Geometry check sheet. Reference: the model listing, model coordinates, mm. Face numbers are marked on the shaded views. Coordinates: 2 decimals unless noted, no trailing zeros. Loops run counter-clockwise (first coordinate to the right, second up) from the corner with the lowest first, then second, coordinate; pieces in that order, holes last. Notation, with made-up numbers: (2.5, -27) -> (61.5, -27) arc R24 ccw to (61.5, 5) -> close; hole circle Ø7 at (7, 57). An arc over 180 degrees is marked (long way). Answer as a JSON object with one key per item and string values.
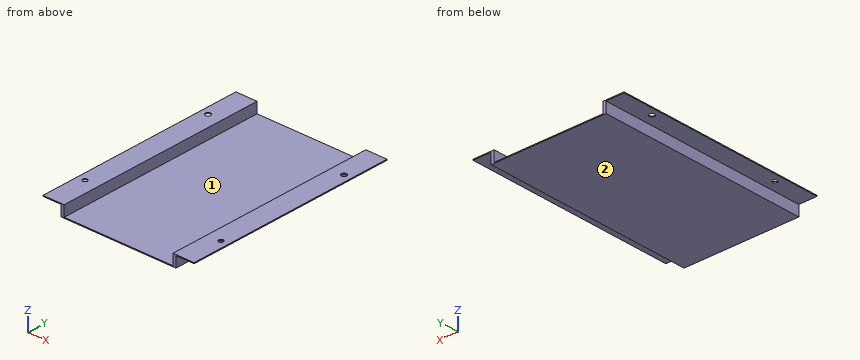
Autodesk Inventor part; units mm, degrees
ref_plane "YZ Plane" through (0, 0, 0) normal (1, 0, 0) x (0, 1, 0)
ref_plane "XZ Plane" through (0, 0, 0) normal (0, 1, 0) x (-1, 0, 0)
ref_plane "XY Plane" through (0, 0, 0) normal (0, 0, 1) x (1, 0, 0)
sketch "Skizze1" plane through (0, 0, 0) normal (0, 0, 1) x (1, 0, 0)
  line L0 (-90, 421.0534) -> (-90, 451.3884) construction
  line L1 (-90, 311.0534) -> (10, 311.0534)
  line L2 (10, 311.0534) -> (10, 451.0534)
  line L3 (10, 451.0534) -> (-90, 451.0534)
  line L4 (-90, 451.0534) -> (-90, 311.0534)
  circle A0 centre (5, 336.0534) radius 1.55
  circle A1 centre (-85, 425.3034) radius 1.75
  line L5 (10, 304.3034) -> (10, 341.0534)
  circle A2 centre (-85, 336.0534) radius 1.55
  circle A3 centre (5, 425.3034) radius 1.75
  line L6 (-90, 304.3034) -> (-90, 341.0534) construction
  point P0 (0, 0)
  dimension "d14" = 25.75
  dimension "d15" = 25
extrude "Extrusion1" add sketch "Skizze1" along normal blind 0.6
sketch "Skizze2" plane through (0, 0, 0) normal (0, 0, -1) x (-1, 0, 0)
  line L0 (90, 311.0534) -> (-10, 311.0534)
  line L1 (-10, 451.0534) -> (90, 451.0534)
  line L2 (2, 311.0534) -> (78, 311.0534)
  line L3 (78, 311.0534) -> (78, 451.0534)
  line L4 (78, 451.0534) -> (2, 451.0534)
  line L5 (2, 451.0534) -> (2, 311.0534)
  line L6 (-10, 311.0534) -> (-10, 451.0534)
  line L7 (90, 451.0534) -> (90, 311.0534)
  line L8 (78, 451.0534) -> (2, 451.0534)
  line L9 (2, 451.0534) -> (2, 311.0534)
  line L10 (2, 311.0534) -> (78, 311.0534)
  line L11 (78, 311.0534) -> (78, 451.0534)
  point P0 (0, 0)
  dimension "d4" = 12
  dimension "d5" = 12
extrude "Extrusion3" add sketch "Skizze2" along normal blind 7 contours L0 L5 L1 L3
sketch "Skizze3" plane through (0, 0, 0.6) normal (0, 0, 1) x (1, 0, 0)
  line L0 (-2, 311.0534) -> (-78, 311.0534) construction
  line L1 (-78, 311.0534) -> (-78, 451.0534) construction
  line L2 (-78, 451.0534) -> (-2, 451.0534) construction
  line L3 (-2, 451.0534) -> (-2, 311.0534) construction
  line L4 (-90, 311.0534) -> (10, 311.0534)
  line L5 (-78, 451.0534) -> (-2, 451.0534)
  line L6 (-4, 311.0534) -> (-76, 311.0534)
  line L7 (-76, 311.0534) -> (-76, 451.0534)
  line L8 (-76, 451.0534) -> (-4, 451.0534)
  line L9 (-4, 451.0534) -> (-4, 311.0534)
  point P0 (0, 0)
  dimension "d10" = 2
  dimension "d11" = 2
extrude "Extrusion4" cut sketch "Skizze3" against normal blind 7
properties part number "PCB-Mount"
1. Section check C-C, the plane y = 352. Record the boundary of the cut face in (x, z).
Evaluation:
{"outline": "(-90, 0) -> (-78, 0) -> (-78, -7) -> (-2, -7) -> (-2, 0) -> (10, 0) -> (10, 0.6) -> (-4, 0.6) -> (-4, -6.4) -> (-76, -6.4) -> (-76, 0.6) -> (-90, 0.6) -> close"}
2. Thickness scan on probe 1 along Y at (x, z) = (5, 0.5); probe 2 along X at (y, z) = (391, -4.75); probe 3 along X at (y, z) = (323.5, 0.25). Record the ranges inside material, lowest first. Write a range as from..to.
Evaluation:
{"probe 1": "y = 311.05..334.5, 337.6..423.55, 427.05..451.05", "probe 2": "x = -78..-76, -4..-2", "probe 3": "x = -90..-76, -4..10"}
3. Section check D-D, the plane x = -27.5. Record the boundary of the cut face in (y, z).
Evaluation:
{"outline": "(311.05, -7) -> (451.05, -7) -> (451.05, -6.4) -> (311.05, -6.4) -> close"}
4. Mould release check, pull along X, two halves, no side actions. Record for the marked faces 1 and 2: released by +X, released by -X, zero draft, split by the parting line, or undercut.
Evaluation:
{"face 1": "undercut", "face 2": "zero draft"}
5. Section check A-A, the plane z = -5.25. Record the boundary of the cut face in (x, y).
Evaluation:
{"outline": "(-78, 311.05) -> (-76, 311.05) -> (-76, 451.05) -> (-78, 451.05) -> close; (-4, 311.05) -> (-2, 311.05) -> (-2, 451.05) -> (-4, 451.05) -> close"}
6. Section check B-B, the plane x = 5. Record the boundary of the cut face in (y, z), then the cut area to 3 significant figures.
Evaluation:
{"outline": "(311.05, 0) -> (334.5, 0) -> (334.5, 0.6) -> (311.05, 0.6) -> close; (337.6, 0) -> (423.55, 0) -> (423.55, 0.6) -> (337.6, 0.6) -> close; (427.05, 0) -> (451.05, 0) -> (451.05, 0.6) -> (427.05, 0.6) -> close", "area": "80.0 mm^2"}
7. Depth check by flat-ended pin: P1, Ø2, axis at y = 404, z = -5, coming from the +X side; P2, Ø2, axis at y = 400, z = -3, coming from the -X side; P3, Ø5.5, axis at x = 5, y = 425.3, coming from the -Z side. Enter the tip coordinate at first touch or a pass-through.
Evaluation:
{"P1": "stops at x = -2", "P2": "stops at x = -78", "P3": "stops at z = 0"}
